from build123d import *

# Parameters (mm, degrees)
CUT_EXTRUDE1_DEPTH  = 14.549134849
BOSS_EXTRUDE1_START = 2
SKETCH5_R           = 9.254000034
BOSS_EXTRUDE1_DEPTH = 2


with BuildPart() as part:
    # Sketch3 → Revolve1 (revolve)
    with BuildSketch(Plane.XY):
        with BuildLine():
            Line((1.753997, 0), (-1.753997, 0))
            Line((-1.753997, 0), (-1.753997, 9.254000034))
            ThreePointArc((-1.753997, 9.254000034), (0, 7.500003034), (1.753997, 9.254000034))
            Line((1.753997, 9.254000034), (1.753997, 0))
        make_face()
    revolve(axis=Axis((1.753997, 0, 0), (-1, 0, 0)))

    # Sketch4 → Cut-Extrude1 (cut, through all)
    with BuildSketch(Plane.ZY.offset(1.753997)):
        with BuildLine():
            Line((0, 3), (-2.645751311, 3))
            ThreePointArc((-2.645751311, 3), (0, -4), (2.645751311, 3))
            Line((2.645751311, 3), (0, 3))
        make_face()
    extrude(amount=-CUT_EXTRUDE1_DEPTH, mode=Mode.SUBTRACT)

    # Sketch5 → Boss-Extrude1 (add)
    with BuildSketch(Plane.ZY.offset(1.753997).offset(BOSS_EXTRUDE1_START)):
        with Locations(Location((0, 0, 0), (0, 0, 270))):
            Circle(SKETCH5_R)
        with BuildLine():
            Line((2.645751311, 3), (-2.645751311, 3))
            ThreePointArc((-2.645751311, 3), (0, -4), (2.645751311, 3))
        make_face(mode=Mode.SUBTRACT)
    boss_extrude1 = extrude(amount=-BOSS_EXTRUDE1_DEPTH)

    # Mirror1: Boss-Extrude1 across plane
    add(boss_extrude1.mirror(Plane(origin=(0, 0, 0), x_dir=(0, 0, 1), z_dir=(1, 0, 0))))


solid = part.part
CAD build for the part. Positions are in the model's coordinates, mm. Give positions to 0.01 mm unless a question says otherwise; leave off trailing zeros. Loops run counter-clockwise (first coordinate to the right, second up) from the corner with the lowest first, then second, coordinate; pieces in that order, holes last. Notation, with made-up numbers: M 83,-34.75 L 134,-34.75 A21 cw 134,-12.75 Z; hole C 68,-37 d2. An arc over 180 degrees is marked long. One line per question, with ' | ' between items. Start each with the question number.
1. Probe L1, parallel to Z at x = 0.75, y = -1; L2, parallel to Y at x = -3, z = -2; L3, parallel to Z at x = -1.5, y = 0. List the from-to ranges inside material, lowest first. Write a range as from..to.
2. Saw through at B-B on z = 0. Give the cut face in (x, y).
3. Saw through at C-C on x = 1.25. Give the cut face in (y, z).
4. Two-plate mould, pull along Z, no slides. Class faces 1 (the face through (-2.768, 7.344, -5.631)), 2 (the face through (3.754, -4, -2)), 3 (the face through (0, 3, 0)): pulls with the +Z half, pulls with the -Z half, needs draft (parallel to the pull), parting line crosses it, or undercut.
5. Saw through at A-A on y = 0. Give the cut face in (x, z).
6. Flat gauge pins, fed straight in: pin 1 (1.6 mm diameter, centred on x = -0.5, z = -0.5, fed in from -Y); pin 2 (4 mm diameter, centred on x = -2, y = 7, fed in from -Z); pin 3 (4 mm diameter, centred on x = 0.5, z = -7, fed in from +Y); pin 4 (10.5 mm diameter, centred on y = 0, z = 0, fed in from -X). Where does each tip first touch, or does it go through?
Result sheet:
1) L1: z = -7.6..-3.87, 3.87..7.6 | L2: y = -9.04..-3.46, 3..9.04 | L3: z = -8.34..-4, 4..8.34
2) outline: M -3.75,-9.25 L -1.75,-9.25 A1.75 cw 1.75,-9.25 L 3.75,-9.25 L 3.75,-4 L -3.75,-4 Z; M -3.75,3 L 3.75,3 L 3.75,9.25 L 1.75,9.25 A1.75 cw -1.75,9.25 L -3.75,9.25 Z
3) outline: C 0,0 d16.05; hole M 3,-2.65 L 3,2.65 A4 ccw long Z
4) face 1: parting line crosses it | face 2: needs draft | face 3: undercut
5) outline: M -3.75,-9.25 L -1.75,-9.25 A1.75 cw 1.75,-9.25 L 3.75,-9.25 L 3.75,-4 L -3.75,-4 Z; M -3.75,4 L 3.75,4 L 3.75,9.25 L 1.75,9.25 A1.75 cw -1.75,9.25 L -3.75,9.25 Z
6) pin 1: stops at y = -8.06 | pin 2: stops at z = -7.79 | pin 3: stops at y = 7.48 | pin 4: stops at x = -3.75
